The listing builds one solid part. Answer for the finished solid, in the listing's coordinates (mm). Face numbers are marked on the shaded views. A direction names the side the tool comes from. Coordinates: 2 decimals unless noted, no trailing zeros. Order: outer loops, then holes, each group sorted by start corner. A loop starts at its lowest first (then second) coordinate and runs counter-clockwise, first axis right, second up.
```python
from build123d import *

# Parameters (mm, degrees)
F0_R     = 15
F1_DEPTH = 1
F1_TAPER = 30
F2_DEPTH = 3
F4_DEPTH = 2
F5_R     = 1.5
F6_DEPTH = 2.001
F7_W     = 13.4332590942
F7_H     = 2
F7_W_2   = 2
F7_H_2   = 13.4332590942
F8_DEPTH = 1
F9_R     = 0.99999


# Not quite as in the source:
# - a fillet or chamfer is up to 0.001 mm smaller than in the source, because OpenCascade refuses the exact size


with BuildPart() as f1:
    # F0 (on Top) → F1 (new body)
    with BuildSketch(Plane.XY):
        Circle(F0_R)
    extrude(amount=F1_DEPTH, taper=F1_TAPER)

    # F2 (add): a face of the model
    f2_faces = [f1.faces().sort_by_distance(p)[0] for p in [
        (0, 0, 1),
    ]]
    extrude(f2_faces, amount=F2_DEPTH)

    # F3 (on face) → F4 (cut)
    with BuildSketch(Plane.XY.offset(4)):
        Polygon((2.8, -1.6165807537), (2.8, 1.6165807537), (0, 3.2331615075), (-2.8, 1.6165807537), (-2.8, -1.6165807537), (0, -3.2331615075), align=None)
    extrude(amount=-F4_DEPTH, mode=Mode.SUBTRACT)

    # F5 (on face) → F6 (cut, through all)
    with BuildSketch(Plane.XY.offset(2)):
        Circle(F5_R)
    extrude(amount=-F6_DEPTH, mode=Mode.SUBTRACT)

    # F7 (on face) → F8 (join)
    with BuildSketch(Plane(origin=(0, 0, 0), x_dir=(1, 0, 0), z_dir=(0, 0, -1))):
        with Locations((-8.25, 0)):
            Rectangle(F7_W, F7_H)
        with Locations((0, 8.25)):
            Rectangle(F7_W_2, F7_H_2)
        with Locations((8.25, 0)):
            Rectangle(F7_W, F7_H)
        with Locations((0, -8.25)):
            Rectangle(F7_W_2, F7_H_2)
    extrude(amount=F8_DEPTH)

    # F9 (radius 1 in the source; OpenCascade refuses exactly that, so slightly less here)
    f9_edges = [f1.edges().sort_by_distance(p)[0] for p in [
        (-1, 8.25, -1),
        (1, 8.25, -1),
        (8.25, 1, -1),
        (14.96663, 0, -1),
        (8.25, -1, -1),
        (1.53337, 0, -1),
        (-8.25, 1, -1),
        (-8.25, -1, -1),
        (1, -8.25, -1),
        (-1, -8.25, -1),
        (0, 14.96663, -1),
        (0, 1.53337, -1),
        (0, -1.53337, -1),
        (-1.53337, 0, -1),
        (-14.96663, 0, -1),
        (0, -14.96663, -1),
    ]]
    fillet(f9_edges, radius=F9_R)


solid = f1.part
```
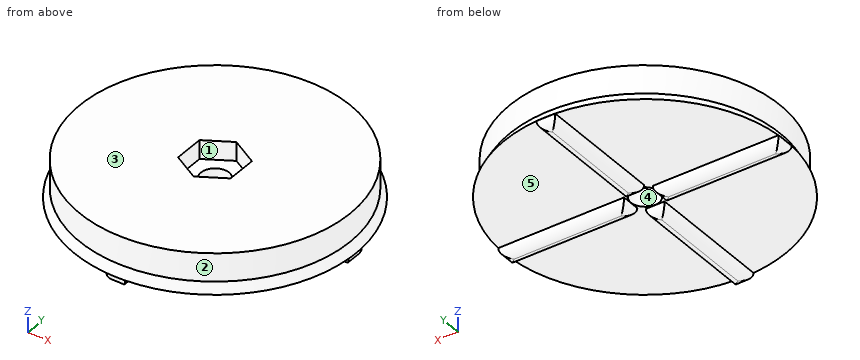
(1) The mould has two halves that part along Y. Classify the marked faces 1, 2 and 3: released by +Y, released by -Y, zero draft, split by the parting line, or undercut.
(2) For the marked faces 4 and 5, determine the directions among +Z, -Z, +X, -X, +Y, -Y from which every point of the face is accessible in a straight line to the end or side of a thin tool.
(3) Each of these flat-tipped pins is pushed along its axis until it touches: pin 1 Ø1.5 at (x, z) = (0, 1) entering from +Y; pin 2 Ø10 at (x, y) = (-7, 7.5) entering from -Z; pin 3 Ø4 at (x, y) = (0, 0) entering from -Z. Where does it stop, or does it pass through?
(4) Consider line 1 (Y direction, x = 0, z = 1.4); line 2 (Z direction, x = 9.5, y = 7); line 3 (Y direction, x = 2, z = -0.1). Determine where each line is inside the solid, lowest interval first.
(5) Find section B-B (z = 2.4). Write down the section's boundary in (x, y), and give its area (3 significant figures).
(6) Find section A-A (z = -0.4). Write down the section's boundary in (x, y), and give its area (3 significant figures).
Findings below:
1. face 1: undercut
1. face 2: split by the parting line
1. face 3: zero draft
2. face 4: +Z, -Z
2. face 5: -Z
3. pin 1: stops at y = 14.86
3. pin 2: stops at z = 0
3. pin 3: stops at z = -0.85
4. line 1: y = -14.42 to -1.5, 1.5 to 14.42
4. line 2: z = 0 to 4
4. line 3: y = -0.99 to 0.99
5. outline: circle Ø28.85 at (0, 0); hole (-2.8, -1.62) - (0, -3.23) - (2.8, -1.62) - (2.8, 1.62) - (0, 3.23) - (-2.8, 1.62) - close
5. area: 626 mm2
6. outline: (-14.88, -0.92) - (-1.62, -0.92) - (-1.62, 0.92) - (-14.88, 0.92) - close; (-0.92, -14.88) - (0.92, -14.88) - (0.92, -1.62) - (-0.92, -1.62) - close; (-0.92, 1.62) - (0.92, 1.62) - (0.92, 14.88) - (-0.92, 14.88) - close; (1.62, -0.92) - (14.88, -0.92) - (14.88, 0.92) - (1.62, 0.92) - close
6. area: 97.3 mm2
